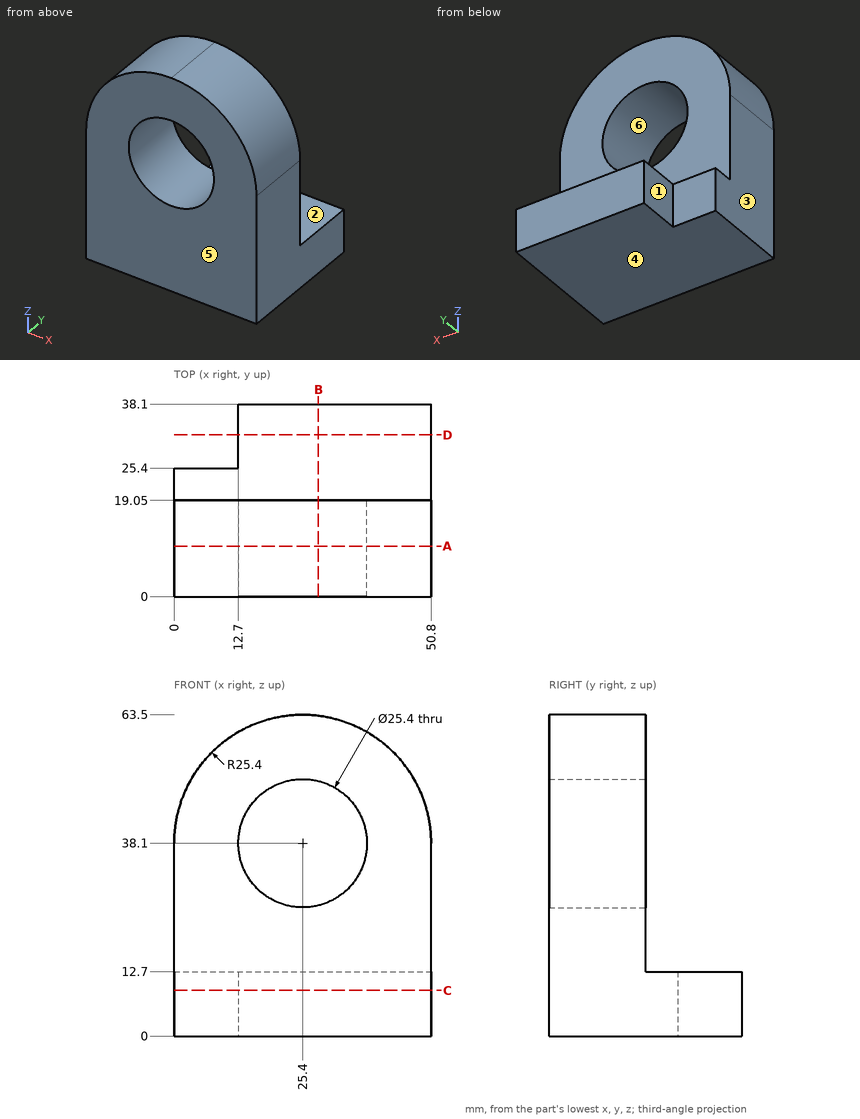
Check sheet for the drawn part. Datum: minimum x, y, z corner. Units: mm. A direction names the side the tool comes from. Give positions to 0.01 mm unless a question says otherwise; leave off trailing zeros. Write each loop counter-clockwise with the first axis right and the second up, starting at its lowest first coordinate (ties: lowest second). Pieces come first, ordered by that corner, then holes.
(1) Cross-section at D-D (y = 32). Enter the section's corners in (x, z), plus the area to 3 significant figures.
(2) Access from +Z, -Z, +X, -X, +Y, -Y to the whole of each face (thin tool, end or side, straight path). Record for the marked faces 1, 2 and 3.
(3) Cross-section at A-A (y = 10). Enter the section's corners in (x, z), plus the area to 3 significant figures.
(4) Cross-section at B-B (x = 28.5). Enter the section's corners in (y, z), plus the area to 3 significant figures.
(5) Gauge pin test, flat ends, axial feed: pin 1 (1.5 mm diameter, centred on x = 8, y = 18, fed in from +Z); pin 2 (12 mm diameter, centred on x = 24.5, y = 33.5, fed in from +Z); pin 3 (15 mm diameter, centred on x = 24.5, z = 25.5, fed in from +Y); pin 4 (23 mm diameter, centred on x = 25.4, z = 38.1, fed in from +Y). Record the tip position at first contact, or that the pin passes through.
(6) Mould release check, pull along Z, two halves, no side actions. Record for the marked faces 4, 5 and 6: +Z half, -Z half, draft (parallel to the pull), parting line (faces both ways), or undercut.
(7) Material ranges on line 1 (Z direction, x = 22, y = 6); line 2 (X direction, y = 14, z = 38); line 3 (Y direction, x = 35, z = 25), recorded low to high.
(8) Cross-section at C-C (z = 9). Enter the section's corners in (x, y), plus the area to 3 significant figures.
Worked out:
1. outline: (12.7, 0) - (50.8, 0) - (50.8, 12.7) - (12.7, 12.7) - close
1. area: 484 mm2
2. face 1: +Z, -Z, -X, +Y
2. face 2: +Z, +X, -X, +Y
2. face 3: +Z, -Z, -X, +Y, -Y
3. outline: (0, 0) - (50.8, 0) - (50.8, 38.1) arc R25.4 ccw to (0, 38.1) - close; hole circle Ø25.4 at (25.4, 38.1)
3. area: 2,440 mm2
4. outline: (0, 0) - (38.1, 0) - (38.1, 12.7) - (19.05, 12.7) - (19.05, 25.78) - (0, 25.78) - close; (0, 50.42) - (19.05, 50.42) - (19.05, 63.31) - (0, 63.31) - close
4. area: 979 mm2
5. pin 1: stops at z = 57.28
5. pin 2: stops at z = 12.7
5. pin 3: stops at y = 19.05
5. pin 4: passes through
6. face 4: -Z half
6. face 5: draft
6. face 6: undercut
7. line 1: z = 0 to 25.86, 50.34 to 63.27
7. line 2: x = 0 to 12.7, 38.1 to 50.8
7. line 3: y = 0 to 19.05
8. outline: (0, 0) - (50.8, 0) - (50.8, 38.1) - (12.7, 38.1) - (12.7, 25.4) - (0, 25.4) - close
8. area: 1,770 mm2
